Read the model definition and answer for the solid it produces. Units are mm, in the model's axes. A direction names the side the tool comes from. Round coordinates to 2 decimals unless told otherwise and drop trailing zeros. Order: outer loops, then holes, each group sorted by start corner. A loop starts at its lowest first (then second) coordinate and runs counter-clockwise, first axis right, second up.
Autodesk Inventor part; units mm, degrees
ref_plane "YZ Plane" through (0, 0, 0) normal (1, 0, 0) x (0, 1, 0)
ref_plane "XZ Plane" through (0, 0, 0) normal (0, 1, 0) x (-1, 0, 0)
ref_plane "XY Plane" through (0, 0, 0) normal (0, 0, 1) x (1, 0, 0)
sketch "Sketch1" plane through (0, 0, 0) normal (0, 1, 0) x (-1, 0, 0)
  line L0 (20, 9.75) -> (-20, 9.75)
  line L1 (-20, 9.75) -> (-20, -9.75)
  line L2 (-20, -9.75) -> (20, -9.75)
  line L3 (20, -9.75) -> (20, 9.75)
  line L4 (20, 9.75) -> (-20, -9.75) construction
  line L5 (-20, 9.75) -> (20, -9.75) construction
  line L6 (21.5, 11.25) -> (-21.5, 11.25)
  line L7 (-21.5, 11.25) -> (-21.5, -11.25)
  line L8 (-21.5, -11.25) -> (21.5, -11.25)
  line L9 (21.5, -11.25) -> (21.5, 11.25)
  line L10 (-20, 11.25) -> (20, 11.25)
  line L11 (20, 11.25) -> (20, -11.25)
  line L12 (20, -11.25) -> (-20, -11.25)
  line L13 (-20, -11.25) -> (-20, 11.25)
  line L14 (-20, 11.25) -> (20, -11.25) construction
  line L15 (20, 11.25) -> (-20, -11.25) construction
  line L16 (25, 14.75) -> (-25, 14.75)
  line L17 (-25, 14.75) -> (-25, -14.75)
  line L18 (-25, -14.75) -> (25, -14.75)
  line L19 (25, -14.75) -> (25, 14.75)
  point P0 (0, 0)
  point P1 (-19.6517, -9.75)
  dimension "d0" = 40
  dimension "d1" = 19.5
  dimension "d2" = 1.5
  dimension "d3" = 3.5
extrude "Extrusion1" add sketch "Sketch1" along normal blind 6 contours L3 L2 L1 L0 | L11 L6 L9 L8 L3 | L1 L13 L8 L7 L6 | L19 L18 L17 L16
fillet "Fillet1" radius 2 12 edges at (0, 6, 14.75) (0, 0, 14.75) (25, 0, 0) (25, 6, 0) (0, 6, -14.75) (0, 0, -14.75) (-25, 0, 0) (-25, 6, 0) (-25, 3, 14.75) (-25, 3, -14.75) (25, 3, -14.75) (25, 3, 14.75)
fillet "Fillet2" radius 0.5 8 edges at (-20, 3, 9.75) (-20, 3, 11.25) (-20, 3, -9.75) (-20, 3, -11.25) (20, 3, -11.25) (20, 3, 9.75) (20, 3, 11.25) (20, 3, -9.75)
fillet "Fillet3" radius 1 32 edges at (-19.8536, 6, -9.8964) (-20, 6, -10.5) (-19.8536, 6, -11.1036) (0, 6, -11.25) (19.8536, 6, -11.1036) (20, 6, -10.5) (19.8536, 6, -9.8964) (0, 6, -9.75) (19.8536, 6, 9.8964) (20, 6, 10.5) (19.8536, 6, 11.1036) (0, 6, 11.25) (-19.8536, 6, 11.1036) (-20, 6, 10.5) (-19.8536, 6, 9.8964) (0, 6, 9.75) (19.8536, 0, 9.8964) (20, 0, 10.5) (19.8536, 0, 11.1036) (0, 0, 11.25) (-19.8536, 0, 11.1036) (-20, 0, 10.5) (-19.8536, 0, 9.8964) (0, 0, 9.75) (-19.8536, 0, -9.8964) (-20, 0, -10.5) (-19.8536, 0, -11.1036) (0, 0, -11.25) (19.8536, 0, -11.1036) (20, 0, -10.5) (19.8536, 0, -9.8964) (0, 0, -9.75)
properties part number "Trimming Template_3DPrint"
Q1. A cutting plane is placed at A-A, the plane x = 6.5. Give the vertices of the cut face in (y, z).
Outcome:
outline: (0, -12.75) arc R2 ccw to (2, -14.75) - (4, -14.75) arc R2 ccw to (6, -12.75) - (6, -12.25) arc R1 ccw to (5, -11.25) - (1, -11.25) arc R1 ccw to (0, -12.25) - close; (0, -8.75) arc R1 ccw to (1, -9.75) - (5, -9.75) arc R1 ccw to (6, -8.75) - (6, 8.75) arc R1 ccw to (5, 9.75) - (1, 9.75) arc R1 ccw to (0, 8.75) - close; (0, 12.25) arc R1 ccw to (1, 11.25) - (5, 11.25) arc R1 ccw to (6, 12.25) - (6, 12.75) arc R2 ccw to (4, 14.75) - (2, 14.75) arc R2 ccw to (0, 12.75) - close
Q2. For a pull along Z with two mould halves and no side action, classify faces 4 (the face through (0.273, 5.715, 9.449)), 5 (the face through (20.285, 0.301, -10.496)), 6 (the face through (-0.32, 0.6, -14.18)), 7 (the face through (0, 3, 14.75)) as released by +Z, released by -Z, zero draft, split by the parting line, or undercut.
Outcome:
face 4: undercut
face 5: undercut
face 6: released by -Z
face 7: released by +Z
Q3. Straight lines are drawn through the part: probe 1 along Z at (x, y) = (-14.5, 2.4); probe 2 along Z at (x, y) = (2, 5.4); probe 3 along X at (y, z) = (4.2, 1.75). For each, find the intervals that lie inside material, in ascending order.
Outcome:
probe 1: z = -14.75 to -11.25, -9.75 to 9.75, 11.25 to 14.75
probe 2: z = -14.18 to -11.33, -9.67 to 9.67, 11.33 to 14.18
probe 3: x = -24.99 to 24.99
Q4. A cutting plane is placed at B-B, the plane y = 2.55. Give the vertices of the cut face in (x, z), plus the area to 3 significant figures.
Outcome:
outline: (-25, -12.75) arc R2 ccw to (-23, -14.75) - (23, -14.75) arc R2 ccw to (25, -12.75) - (25, 12.75) arc R2 ccw to (23, 14.75) - (-23, 14.75) arc R2 ccw to (-25, 12.75) - close; hole (-20, -10.75) arc R0.5 ccw to (-19.5, -11.25) - (19.5, -11.25) arc R0.5 ccw to (20, -10.75) - (20, -10.25) arc R0.5 ccw to (19.5, -9.75) - (-19.5, -9.75) arc R0.5 ccw to (-20, -10.25) - close; hole (-20, 10.25) arc R0.5 ccw to (-19.5, 9.75) - (19.5, 9.75) arc R0.5 ccw to (20, 10.25) - (20, 10.75) arc R0.5 ccw to (19.5, 11.25) - (-19.5, 11.25) arc R0.5 ccw to (-20, 10.75) - close
area: 1,350 mm2
Q5. For faces 1 (the face through (-20.285, 0.301, -10.504)), 2 (the face through (20.301, 5.715, -10.496)), 3 (the face through (0, 3, 11.25)), determine the directions among +Z, -Z, +X, -X, +Y, -Y from which every point of the face is accessible in a straight line to the end or side of a thin tool.
Outcome:
face 1: -Y
face 2: +Y
face 3: +Y, -Y
